Geometry: see drawing. Coordinates: mm, zero at the bounding-box minimum. A direction names the side the tool comes from. Round coordinates to 2 decimals unless told otherwise and drop trailing zeros. Write each loop counter-clockwise with the first axis right and the second up, starting at its lowest first coordinate (ties: lowest second). Pieces come first, ordered by that corner, then holes. Notation, with made-up numbers: M 14,-26.75 L 40,-26.75 A27 cw 40,-1.75 Z; hole C 55,-5 d8. An arc over 180 degrees is marked long. Use one line per item in the form item = value. Start each with the question number.
Item 1: Ray query, probe 1 along Y at (x, z) = (7.62, 4.25); probe 2 along Z at (x, y) = (2, 3.5); probe 3 along Z at (x, y) = (12, 5.25). Return the intervals inside material, ascending.
Item 2: Pull-direction query (Z, two-part tool) for the marked faces 1, 2 and 3; classes: pulls with the +Z half, pulls with the -Z half, needs draft (parallel to the pull), parting line crosses it, or undercut.
Item 3: Section query D-D (y = 3). Return loops of the section in (x, z) (1 decimal), and give its area (3 significant figures).
Item 4: Section query A-A (x = 7.62). Return loops of the section in (y, z).
Item 5: Pin query (flat end, axial travel): pin 1 Ø4 at (y, z) = (12.5, 3.5) entering from +X; pin 2 Ø2 at (x, z) = (9, 6.5) entering from +Y; pin 3 Ø3 at (y, z) = (7, 8) entering from +X. Return the tip coordinate at first contact, or that it passes through.
Item 6: Reachability of the marked faces 4, 5 and 6 from +Z, -Z, +X, -X, +Y, -Y: full face, straight path, thin tool, end or side. Return the list, or none.
Item 7: Section query B-B (z = 6.5). Return loops of the section in (x, y).
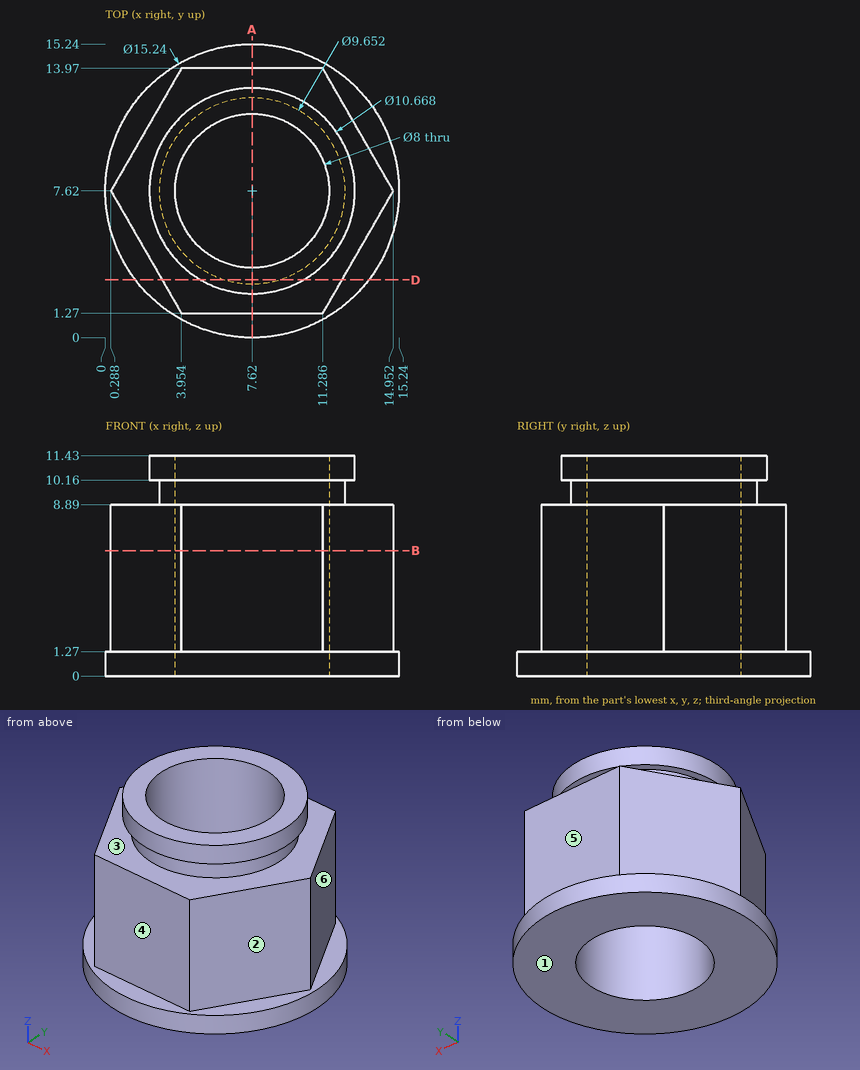
Working result:
q1.probe_1 = 1.27 to 3.62, 11.62 to 13.97
q1.probe_2 = 0 to 1.27
q1.probe_3 = 0 to 8.89, 10.16 to 11.43
q2.face_1 = pulls with the -Z half
q2.face_2 = needs draft
q2.face_3 = undercut
q3.outline = M 1.6,0 L 13.7,0 L 13.7,1.3 L 12.3,1.3 L 12.3,8.9 L 9,8.9 L 9,10.2 L 10.3,10.2 L 10.3,11.4 L 5,11.4 L 5,10.2 L 6.2,10.2 L 6.2,8.9 L 3,8.9 L 3,1.3 L 1.6,1.3 Z
q3.area = 96.8 mm²
q4.outline = M 0,0 L 3.62,0 L 3.62,11.43 L 2.29,11.43 L 2.29,10.16 L 2.79,10.16 L 2.79,8.89 L 1.27,8.89 L 1.27,1.27 L 0,1.27 Z; M 11.62,0 L 15.24,0 L 15.24,1.27 L 13.97,1.27 L 13.97,8.89 L 12.45,8.89 L 12.45,10.16 L 12.95,10.16 L 12.95,11.43 L 11.62,11.43 Z
q5.pin_1 = 13.29
q5.pin_2 = 13.97
q5.pin_3 = 14.95
q6.face_4 = +Z, +X, -X, -Y
q6.face_5 = +Z, +X, -X, +Y
q6.face_6 = +Z, +X, +Y
q7.outline = M 0.29,7.62 L 3.95,1.27 L 11.29,1.27 L 14.95,7.62 L 11.29,13.97 L 3.95,13.97 Z; hole C 7.62,7.62 d8
